Work out the finished part from the listing and answer in its coordinate system (mm). Face numbers are marked on the shaded views. A direction names the side the tool comes from. Round coordinates to 2 decimals unless told otherwise and drop trailing zeros. Order: outer loops, then holes, each group sorted by start corner. A loop starts at its lowest first (then second) coordinate and runs counter-clockwise, first axis right, second up. Notation, with made-up numbers: (-19.5, 89) - (16.5, 89) arc R22 ccw to (16.5, 111) - close; hole circle Ø5 at (70, -24). An arc over 180 degrees is marked (long way). One line per question, with ' | ' between items. Start each with the question number.
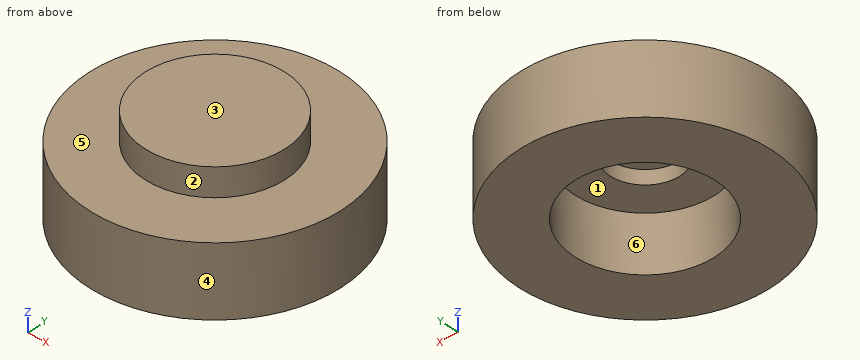
from build123d import *

# Parameters (mm, degrees)
SKETCH_1_R          = 45
EXTRUDE_1_DEPTH     = 35
SKETCH_4_R          = 12.5
CUT_EXTRUDE_3_DEPTH = 25
CUT_EXTRUDE_START   = -10
SKETCH_5_R          = 45
SKETCH_5_R_2        = 25
CUT_EXTRUDE_4_DEPTH = 10
SKETCH_6_R          = 25
CUT_EXTRUDE_6_DEPTH = 20


with BuildPart() as part:
    # Эскиз1 → Вытянуть1 (new body)
    with BuildSketch(Plane.XY):
        Circle(SKETCH_1_R)
    extrude(amount=EXTRUDE_1_DEPTH)

    # Эскиз4 → Вытянуть3 (cut)
    with BuildSketch(Plane(origin=(0, 0, 0), x_dir=(-1, 0, 0), z_dir=(0, 0, -1))):
        Circle(SKETCH_4_R)
    extrude(amount=-CUT_EXTRUDE_3_DEPTH, mode=Mode.SUBTRACT)

    # Эскиз5 → Вытянуть4 (cut)
    with BuildSketch(Plane.XY.offset(35).offset(CUT_EXTRUDE_START)):
        Circle(SKETCH_5_R)
        Circle(SKETCH_5_R_2, mode=Mode.SUBTRACT)
    extrude(amount=CUT_EXTRUDE_4_DEPTH, mode=Mode.SUBTRACT)

    # Эскиз6 → Вытянуть6 (cut)
    with BuildSketch(Plane(origin=(0, 0, 0), x_dir=(-1, 0, 0), z_dir=(0, 0, -1))):
        with Locations(Location((0, 0, 0), (0, 0, 180))):
            Circle(SKETCH_6_R)
    extrude(amount=-CUT_EXTRUDE_6_DEPTH, mode=Mode.SUBTRACT)


solid = part.part
1) Determine the mould class of the marked faces 4, 5 and 6 for opening direction X: released by +X, released by -X, zero draft, split by the parting line, or undercut.
2) Flat-ended cylindrical pins translate along their axes: pin 1 (4 mm diameter, centred on y = 9, z = 22.5, fed in from -X); pin 2 (1.5 mm diameter, centred on y = -25.5, z = 16.5, fed in from -X); pin 3 (1.5 mm diameter, centred on y = 9.5, z = 15.5, fed in from -X). Find the tip coordinate at first contact, or state that the pin passes through.
3) Straight lines are drawn through the part: line 1 (Y direction, x = 0, z = 23); line 2 (Y direction, x = 0, z = 8); line 3 (Z direction, x = -19.5, y = 40). For each, find the intervals that lie inside material, in ascending order.
4) Section C-C on z = 9 is taken. Give the vertices of the cut face in (x, y).
5) For the marked faces 1, 2 and 3, determine the directions among +Z, -Z, +X, -X, +Y, -Y from which every point of the face is accessible in a straight line to the end or side of a thin tool.
6) Section D-D on x = -22 is taken. Give the vertices of the cut face in (y, z).
7) Section A-A on y = 0 is taken. Give the vertices of the cut face in (x, z), and give its area (4 significant figures).
Recorded:
1) face 4: split by the parting line | face 5: zero draft | face 6: undercut
2) pin 1: stops at x = -44.45 | pin 2: stops at x = -37.58 | pin 3: stops at x = -44.14
3) line 1: y = -45 to -12.5, 12.5 to 45 | line 2: y = -45 to -25, 25 to 45 | line 3: z = 0 to 25
4) outline: circle Ø90 at (0, 0); hole circle Ø50 at (0, 0)
5) face 1: -Z | face 2: +Z | face 3: +Z, +X, -X, +Y, -Y
6) outline: (-39.26, 0) - (-11.87, 0) - (-11.87, 20) - (11.87, 20) - (11.87, 0) - (39.26, 0) - (39.26, 25) - (11.87, 25) - (11.87, 35) - (-11.87, 35) - (-11.87, 25) - (-39.26, 25) - close
7) outline: (-45, 0) - (-25, 0) - (-25, 20) - (-12.5, 20) - (-12.5, 25) - (12.5, 25) - (12.5, 20) - (25, 20) - (25, 0) - (45, 0) - (45, 25) - (25, 25) - (25, 35) - (-25, 35) - (-25, 25) - (-45, 25) - close | area: 1,625 mm²
